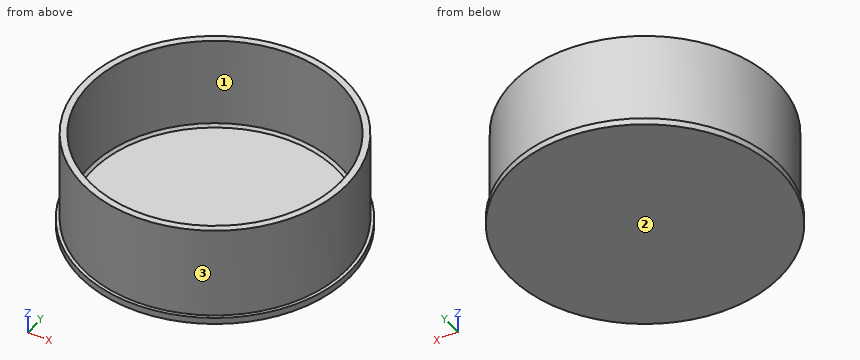
```python
from build123d import *

# Parameters (mm, degrees)
SKETCH_R      = 102.5
PAD_DEPTH     = 5
SKETCH001_R   = 100
SKETCH001_R_2 = 95
PAD001_DEPTH  = 70
CHAMFER_SIZE  = 2


with BuildPart() as part:
    # Sketch → Pad (new body)
    with BuildSketch(Plane.XY):
        Circle(SKETCH_R)
    extrude(amount=PAD_DEPTH)

    # Sketch001 (on DatumPlane) → Pad001 (join)
    with BuildSketch(Plane.XY.offset(5)):
        Circle(SKETCH001_R)
        Circle(SKETCH001_R_2, mode=Mode.SUBTRACT)
    extrude(amount=PAD001_DEPTH)

    # Chamfer
    chamfer_edges = [part.edges().sort_by_distance(p)[0] for p in [
        (-95, 0, 5),
    ]]
    chamfer(chamfer_edges, length=CHAMFER_SIZE)


solid = part.part
```
Read the model definition and answer for the solid it produces. Units are mm, in the model's axes. Face numbers are marked on the shaded views. Give positions to 0.01 mm unless a question says otherwise; leave off trailing zeros. Write each loop counter-clockwise with the first axis right and the second up, starting at its lowest first coordinate (ties: lowest second). Pieces come first, ordered by that corner, then holes. Notation, with made-up numbers: (30.5, 61.25) -> (62.5, 61.25) arc R13 ccw to (62.5, 65.25) -> close; hole circle Ø3 at (-4, -33). An arc over 180 degrees is marked (long way). Answer in a Markdown table with one row per item.
1) Section C-C on z = 59 is taken. Give the vertices of the cut face in (x, y), plus the area to 3 significant figures.
Results list:
| item | result |
|---|---|
| outline | circle Ø200 at (0, 0); hole circle Ø190 at (0, 0) |
| area | 3,060 mm^2 |
2) Section A-A on y = 0 is taken. Give the vertices of the cut face in (x, z).
Results list:
| item | result |
|---|---|
| outline | (-102.5, 0) -> (102.5, 0) -> (102.5, 5) -> (100, 5) -> (100, 75) -> (95, 75) -> (95, 7) -> (93, 5) -> (-93, 5) -> (-95, 7) -> (-95, 75) -> (-100, 75) -> (-100, 5) -> (-102.5, 5) -> close |
3) Each of these flat-tipped pins is pushed along its axis until it touches: pin 1 Ø1.5 at (y, z) = (-29.5, 12.5) entering from +X; pin 2 Ø12 at (y, z) = (-28.5, 54.5) entering from +X; pin 3 Ø8 at (x, z) = (-34.5, 65) entering from +Y; pin 4 Ø12 at (x, y) = (-39.5, -32) entering from -Z. Where does it stop, or does it pass through?
Results list:
| item | result |
|---|---|
| pin 1 | x = 95.78 |
| pin 2 | x = 97.44 |
| pin 3 | y = 95.24 |
| pin 4 | z = 0 |
4) Determine the mould class of the marked faces 1, 2 and 3 for opening direction Y: released by +Y, released by -Y, zero draft, split by the parting line, or undercut.
Results list:
| item | result |
|---|---|
| face 1 | undercut |
| face 2 | zero draft |
| face 3 | split by the parting line |
5) Straight lines are drawn through the part: line 1 (Y direction, x = 0, z = 23); line 2 (Z direction, x = 11, y = -14); line 3 (Y direction, x = -21.5, z = 15.5). For each, find the intervals that lie inside material, in ascending order. Write a range as [from, to].
Results list:
| item | result |
|---|---|
| line 1 | [-100, -95], [95, 100] |
| line 2 | [0, 5] |
| line 3 | [-97.66, -92.54], [92.54, 97.66] |
